```python
from build123d import *

# Parameters (mm, degrees)
F0_W      = 76.2
F0_H      = 25.4
F1_DEPTH  = 11.43
F2_R      = 3.81
F3_DEPTH  = 6.35
F4_W      = 76.2
F4_H      = 11.43
F5_DEPTH  = 25.4
F6_W      = 76.2
F6_H      = 25.4
F7_DEPTH  = 9.525
F8_W      = 76.2
F8_H      = 20.955
F9_DEPTH  = 25.4
F10_W     = 76.2
F10_H     = 25.4
F11_DEPTH = 9.525
F12_R     = 3.81
F13_DEPTH = 5.08
F14_R     = 3.81
F15_DEPTH = 6.35


with BuildPart() as f1:
    # F0 (on Top) → F1 (new body)
    with BuildSketch(Plane.XY):
        with Locations((38.1, 12.7)):
            Rectangle(F0_W, F0_H)
    extrude(amount=F1_DEPTH)

    # F2 (on face) → F3 (cut)
    with BuildSketch(Plane.XY.offset(11.43)):
        with Locations((12.7, 12.7)):
            Circle(F2_R)
        with Locations((38.1, 12.7)):
            Circle(F2_R)
        with Locations((63.5, 12.7)):
            Circle(F2_R)
    extrude(amount=-F3_DEPTH, mode=Mode.SUBTRACT)

    # F4 (on face) → F5 (join)
    with BuildSketch(Plane(origin=(0, 25.4, 0), x_dir=(-1, 0, 0), z_dir=(0, 1, 0))):
        with Locations((-38.1, 5.715)):
            Rectangle(F4_W, F4_H)
    extrude(amount=F5_DEPTH)

    # F6 (on face) → F7 (join)
    with BuildSketch(Plane.XY.offset(11.43)):
        with Locations((38.1, 38.1)):
            Rectangle(F6_W, F6_H)
    extrude(amount=F7_DEPTH)

    # F8 (on face) → F9 (join)
    with BuildSketch(Plane(origin=(0, 50.8, 0), x_dir=(-1, 0, 0), z_dir=(0, 1, 0))):
        with Locations((-38.1, 10.4775)):
            Rectangle(F8_W, F8_H)
    extrude(amount=F9_DEPTH)

    # F10 (on face) → F11 (join)
    with BuildSketch(Plane.XY.offset(20.955)):
        with Locations((38.1, 63.5)):
            Rectangle(F10_W, F10_H)
    extrude(amount=F11_DEPTH)

    # F12 (on face) → F13 (cut)
    with BuildSketch(Plane.XY.offset(20.955)):
        with Locations((12.7, 38.1)):
            Circle(F12_R)
        with Locations((38.1, 38.1)):
            Circle(F12_R)
        with Locations((63.5, 38.1)):
            Circle(F12_R)
    extrude(amount=-F13_DEPTH, mode=Mode.SUBTRACT)

    # F14 (on face) → F15 (cut)
    with BuildSketch(Plane.XY.offset(30.48)):
        with Locations((12.7, 63.5)):
            Circle(F14_R)
        with Locations((38.1, 63.5)):
            Circle(F14_R)
        with Locations((63.5, 63.5)):
            Circle(F14_R)
    extrude(amount=-F15_DEPTH, mode=Mode.SUBTRACT)


solid = f1.part
```
For this review, take the finished solid that the model builds, in its own axes (mm). A direction names the side the tool comes from. Round coordinates to 2 decimals unless told otherwise and drop trailing zeros. Write each loop counter-clockwise with the first axis right and the second up, starting at its lowest first coordinate (ties: lowest second). Pieces come first, ordered by that corner, then holes.
1) Take a section at B-B on x = 69. Give the boundary of the cut face in (y, z) (3 decimals).
Answer below:
outline: (0, 0) - (76.2, 0) - (76.2, 30.48) - (50.8, 30.48) - (50.8, 20.955) - (25.4, 20.955) - (25.4, 11.43) - (0, 11.43) - close
2) Take a section at C-C on y = 63.5. Give the boundary of the cut face in (x, z).
Answer below:
outline: (0, 0) - (76.2, 0) - (76.2, 30.48) - (67.31, 30.48) - (67.31, 24.13) - (59.69, 24.13) - (59.69, 30.48) - (41.91, 30.48) - (41.91, 24.13) - (34.29, 24.13) - (34.29, 30.48) - (16.51, 30.48) - (16.51, 24.13) - (8.89, 24.13) - (8.89, 30.48) - (0, 30.48) - close
3) Take a section at D-D on x = 12.7. Give the boundary of the cut face in (y, z) (3 decimals), then the cut area to 3 significant figures.
Answer below:
outline: (0, 0) - (76.2, 0) - (76.2, 30.48) - (67.31, 30.48) - (67.31, 24.13) - (59.69, 24.13) - (59.69, 30.48) - (50.8, 30.48) - (50.8, 20.955) - (41.91, 20.955) - (41.91, 15.875) - (34.29, 15.875) - (34.29, 20.955) - (25.4, 20.955) - (25.4, 11.43) - (16.51, 11.43) - (16.51, 5.08) - (8.89, 5.08) - (8.89, 11.43) - (0, 11.43) - close
area: 1,460 mm2
4) Insertion check: pin 1 Ø5 at (x, y) = (50.5, 52) entering from -Z; pin 2 Ø12 at (x, y) = (63.5, 38.1) entering from +Z (3 decimals); pin 3 Ø6 at (x, y) = (38.1, 38.1) entering from +Z (3 decimals); pin 4 Ø8.5 at (x, y) = (12.5, 11.5) entering from +Z. Each pin has a flat end and moves straight along its axis. Give the tip position at first contact, or say it passes through.
Answer below:
pin 1: stops at z = 0
pin 2: stops at z = 20.955
pin 3: stops at z = 15.875
pin 4: stops at z = 11.43
5) For line 1 along X through (y, z) = (38.5, 17.5); line 2 along X through (y, z) = (60, 29); line 3 along Y through (x, z) = (12.7, 6.75), list the stretches that pass through material, from the lowest coordinate up.
Answer below:
line 1: x = 0 to 8.91, 16.49 to 34.31, 41.89 to 59.71, 67.29 to 76.2
line 2: x = 0 to 11.19, 14.21 to 36.59, 39.61 to 61.99, 65.01 to 76.2
line 3: y = 0 to 8.89, 16.51 to 76.2
6) Mouldability with a two-part tool opening along Y and no side actions: class faces 4 (the face through (63, 64, 24.13)), 5 (the face through (39, 38, 0)), 6 (the face through (38, 25.4, 16)), 7 (the face through (38, 76.2, 15)) as +Y half, -Y half, draft (parallel to the pull), parting line (faces both ways), or undercut.
Answer below:
face 4: undercut
face 5: draft
face 6: -Y half
face 7: +Y half
7) Machinability: for faces 1 (the face through (39, 32, 20.955)), 2 (the face through (62.67, 59.78, 27.35)), 3 (the face through (38, 69, 30.48)), which of the approach directions +Z, -Z, +X, -X, +Y, -Y give a long, thin tool a straight path to every point of the face, cutting with its end or side? Answer none if there is none.
Answer below:
face 1: +Z, +X, -X, -Y
face 2: +Z
face 3: +Z, +X, -X, +Y, -Y
8) Take a section at A-A on z = 27. Give the boundary of the cut face in (x, y), then the cut area to 3 significant figures.
Answer below:
outline: (0, 50.8) - (76.2, 50.8) - (76.2, 76.2) - (0, 76.2) - close; hole circle Ø7.62 at (12.7, 63.5); hole circle Ø7.62 at (38.1, 63.5); hole circle Ø7.62 at (63.5, 63.5)
area: 1,800 mm2
